Source: three-view drawing plus pictorial views. Frame: mm from the lowest corner of the part. A direction names the side the tool comes from. Give positions to 0.01 mm unless a question says otherwise; leave off trailing zeros. Loops run counter-clockwise (first coordinate to the right, second up) from the corner with the lowest first, then second, coordinate; pieces in that order, holes last.
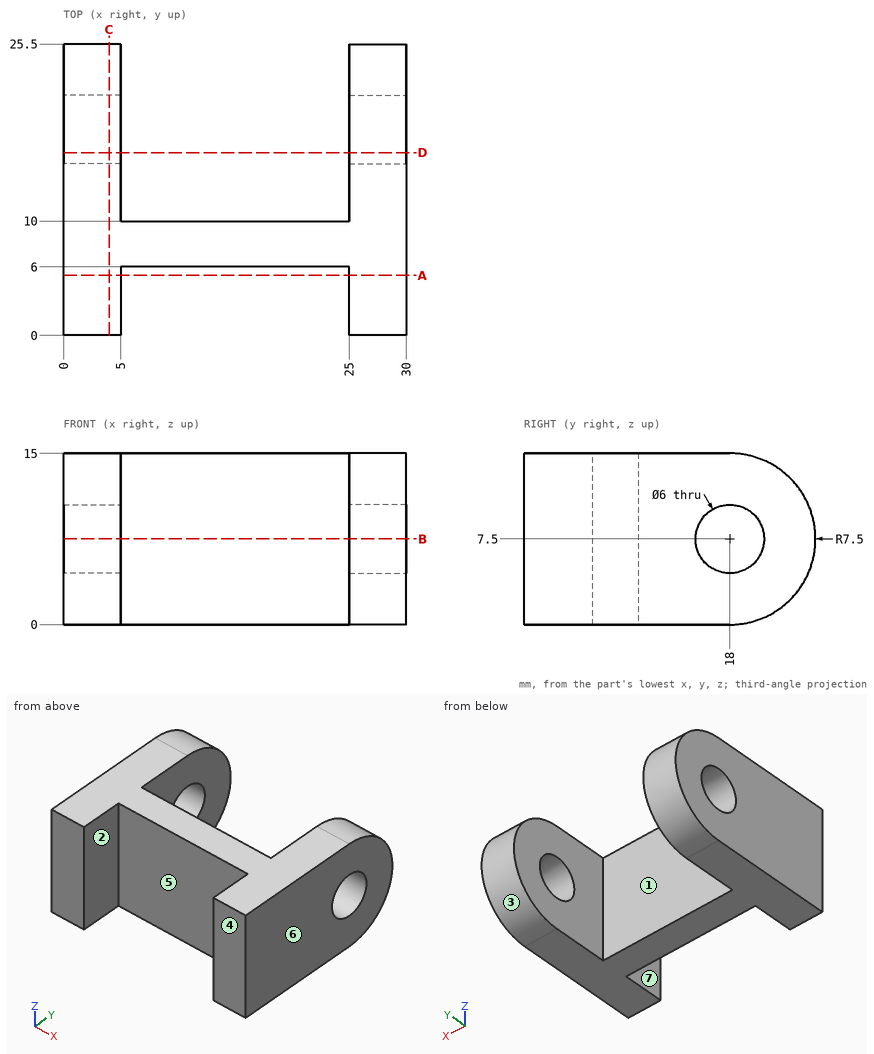
1) Cut plane C-C (x = 4). Return loops of the section in (y, z), and give its area (3 significant figures).
Checks:
outline: (0, 0) - (18, 0) arc R7.5 ccw to (18, 15) - (0, 15) - close; hole circle Ø6 at (18, 7.5)
area: 330 mm2
2) Ray query, probe 1 along Y at (x, z) = (1.9, 7.5); probe 2 along X at (y, z) = (13.75, 12.75); probe 3 along Y at (x, z) = (20.5, 14.5). Return the intervals inside material, ascending.
Checks:
probe 1: y = 0 to 15, 21 to 25.5
probe 2: x = 0 to 5, 25 to 30
probe 3: y = 6 to 10
3) Contact query for flat-ended pins moving along their axis: P1, Ø8, axis at x = 26, z = 8, coming from the +Y side; P2, Ø1.5, axis at x = 23, z = 6.5, coming from the +Y side; P3, Ø7.5, axis at x = 19.5, z = 7, coming from the -Y side; P4, Ø2, axis at x = 3.5, y = 20, coming from the -Z side. Output: stop coordinate, or through.
Checks:
P1: stops at y = 25.5
P2: stops at y = 10
P3: stops at y = 6
P4: stops at z = 0.07
4) Reachability of the marked faces 1, 2 and 3 from +Z, -Z, +X, -X, +Y, -Y: full face, straight path, thin tool, end or side. Return the list, or none.
Checks:
face 1: +Z, -Z, +Y
face 2: +Z, -Z, -Y
face 3: +X, -X, +Y
5) Cut plane D-D (y = 16). Return loops of the section in (x, z), and give its area (3 significant figures).
Checks:
outline: (0, 0) - (5, 0) - (5, 5.26) - (0, 5.26) - close; (0, 9.74) - (5, 9.74) - (5, 15) - (0, 15) - close; (25, 0) - (30, 0) - (30, 5.26) - (25, 5.26) - close; (25, 9.74) - (30, 9.74) - (30, 15) - (25, 15) - close
area: 105 mm2
6) Cut plane A-A (y = 5.25). Return loops of the section in (x, z).
Checks:
outline: (0, 0) - (5, 0) - (5, 15) - (0, 15) - close; (25, 0) - (30, 0) - (30, 15) - (25, 15) - close
7) Pull-direction query (X, two-part tool) for the marked faces 4, 5, 6 and 7; classes: released by +X, released by -X, zero draft, split by the parting line, or undercut.
Checks:
face 4: zero draft
face 5: undercut
face 6: released by +X
face 7: undercut
8) Cut plane B-B (z = 7.5). Return loops of the section in (x, y), and give its area (3 significant figures).
Checks:
outline: (0, 0) - (5, 0) - (5, 6) - (25, 6) - (25, 0) - (30, 0) - (30, 15) - (25, 15) - (25, 10) - (5, 10) - (5, 15) - (0, 15) - close; (0, 21) - (5, 21) - (5, 25.5) - (0, 25.5) - close; (25, 21) - (30, 21) - (30, 25.5) - (25, 25.5) - close
area: 275 mm2
